```python
from build123d import *

# Parameters (mm, degrees)
F1_DEPTH = 3.175
F2_W     = 7.62
F2_H     = 50.8
F3_DEPTH = 12.7
F4_R     = 25.4
F5_R     = 5.08


with BuildPart() as f1:
    # F0 (on Front) → F1 (new body, symmetric)
    with BuildSketch(Plane.XZ):
        Polygon((129.848452, 101.6), (-129.848452, 101.6), (-125.4125, 0), (125.4125, 0), align=None)
    extrude(amount=F1_DEPTH, both=True)

    # F2 (on Front) → F3 (cut, symmetric)
    with BuildSketch(Plane.XZ):
        with Locations((-40.64, 76.2)):
            Rectangle(F2_W, F2_H)
        with Locations((40.64, 76.2)):
            Rectangle(F2_W, F2_H)
    extrude(amount=F3_DEPTH, both=True, mode=Mode.SUBTRACT)

    # F4
    f4_edges = [f1.edges().sort_by_distance(p)[0] for p in [
        (-125.4125, 0, 0),
        (125.4125, 0, 0),
    ]]
    fillet(f4_edges, radius=F4_R)

    # F5
    f5_edges = [f1.edges().sort_by_distance(p)[0] for p in [
        (-129.848452, 0, 101.6),
        (129.848452, 0, 101.6),
    ]]
    fillet(f5_edges, radius=F5_R)


solid = f1.part
```
Work out the finished part from the listing and answer in its coordinate system (mm). A direction names the side the tool comes from. Round coordinates to 2 decimals unless told otherwise and drop trailing zeros. Write each loop counter-clockwise with the first axis right and the second up, starting at its lowest first coordinate (ties: lowest second). Pieces come first, ordered by that corner, then holes.
1) A cutting plane is placed at C-C on z = 71. Determine the outline of the cut face in (x, y) (3 decimals).
2) A cutting plane is placed at A-A on z = 59. Give the number of separate pieces and of enclosed holes in the cut face, and give its area (3 significant figures).
3) A cutting plane is placed at D-D on x = -111. Determine the outline of the cut face in (y, z) (3 decimals), and give its area (3 significant figures).
4) A cutting plane is placed at B-B on y = 1. Determine the outline of the cut face in (x, z).
5) Flat-ended cylindrical pins translate along their axes: P1, Ø2, axis at x = -62, y = -0.5, coming from the -Z side; P2, Ø1.5, axis at y = 1.5, z = 89, coming from the -X side; P3, Ø1.5, axis at y = 0, z = 19, coming from the -X side; P4, Ø1, axis at y = 0.5, z = 43, coming from the -X side. Find the tip coordinate at first contact, or state that the pin passes through.
6) Consider probe 1 along X at (y, z) = (-2.25, 96.5); probe 2 along X at (y, z) = (-2.25, 74.5); probe 3 along X at (y, z) = (2.75, 15.5). Determine where each line is inside the solid, lowest interval first.
7) Determine the mould class of faces 1 (the face through (118.857, 0.044, 7.241)), 2 (the face through (44.45, 0, 76)), 3 (the face through (-36.83, 0, 76)), 4 (the face through (1, 0, 101.6)) for opening direction X: pulls with the +X half, pulls with the -X half, needs draft (parallel to the pull), parting line crosses it, or undercut.
8) Which of the six approach directions +Z, -Z, +X, -X, +Y, -Y give full straight-line access (tool end or side, diameter ignored) to faces 5 (the face through (-84, 0, 101.6)), 6 (the face through (-41, 0, 50.8))?
Entries:
1. outline: (-128.512, -3.175) - (-44.45, -3.175) - (-44.45, 3.175) - (-128.512, 3.175) - close; (-36.83, -3.175) - (36.83, -3.175) - (36.83, 3.175) - (-36.83, 3.175) - close; (44.45, -3.175) - (128.512, -3.175) - (128.512, 3.175) - (44.45, 3.175) - close
2. separate pieces: 3
2. enclosed holes: 0
2. area: 1,530 mm2
3. outline: (-3.175, 2.01) - (3.175, 2.01) - (3.175, 101.6) - (-3.175, 101.6) - close
3. area: 632 mm2
4. outline: (-129.62, 96.3) - (-126.47, 24.29) arc R25.4 ccw to (-101.1, 0) - (101.1, 0) arc R25.4 ccw to (126.47, 24.29) - (129.62, 96.3) arc R5.08 ccw to (124.54, 101.6) - (44.45, 101.6) - (44.45, 50.8) - (36.83, 50.8) - (36.83, 101.6) - (-36.83, 101.6) - (-36.83, 50.8) - (-44.45, 50.8) - (-44.45, 101.6) - (-124.54, 101.6) arc R5.08 ccw to start
5. P1: stops at z = 0
5. P2: stops at x = -129.33
5. P3: stops at x = -125.86
5. P4: stops at x = -127.31
6. probe 1: x = -129.62 to -44.45, -36.83 to 36.83, 44.45 to 129.62
6. probe 2: x = -128.67 to -44.45, -36.83 to 36.83, 44.45 to 128.67
6. probe 3: x = -124.49 to 124.49
7. face 1: pulls with the +X half
7. face 2: undercut
7. face 3: undercut
7. face 4: needs draft
8. face 5: +Z, +X, -X, +Y, -Y
8. face 6: +Z, +Y, -Y
